Design review of the part built by this model. Coordinates are the model's own, in mm. A direction names the side the tool comes from. Give positions to 0.01 mm unless a question says otherwise; leave off trailing zeros. Order: outer loops, then holes, each group sorted by start corner. A loop starts at its lowest first (then second) coordinate and runs counter-clockwise, first axis right, second up. Notation, with made-up numbers: (-10, 40.5) -> (23, 40.5) arc R20 ccw to (23, 70.5) -> close; hole circle Ø8 at (60.5, 77). An arc over 180 degrees is marked (long way). One line per item, written item: value. Start each with the question number.
1) Consider section A-A (x = -49.5). State the section outline as (y, z) points, plus the area to 3 significant figures.
2) Consider section D-D (z = -28). State the section outline as (x, y) points.
3) For pin 1 (0.8 mm diameter, centred on x = -22.5, y = 1, fed in from +Z); pin 2 (0.8 mm diameter, centred on x = -45.5, y = 1, fed in from +Z); pin 3 (0.8 mm diameter, centred on x = -64.5, y = 0.5, fed in from -Z), all flat-tipped, find the tip position at first contact; note any pin that passes through.
4) Consider section C-C (z = -8). State the section outline as (x, y) points, plus the area to 3 significant figures.
5) Tool access review of faces 5 (the face through (-57, 1, -23.7)), 6 (the face through (-21.63, 0.811, -25.415)), 7 (the face through (-58, 1, -25.7)): name each direction out of +Z, -Z, +X, -X, +Y, -Y from which nothing blocks a thin tool from reaching the whole face with its end or side.
6) Wall thickness on line 1 along X through (y, z) = (1, -22); line 2 along Z through (x, y) = (-25, 0.45); line 3 along X through (y, z) = (0.1, 1): over which ranges is each line inside the solid? List them lowest first. Write a range as from..to.
7) Consider section B-B (z = -20.5). State the section outline as (x, y) points.
8) The part is to be moulded in two halves that separate along Z. For faces 1 (the face through (-68.93, 1, -13)), 2 (the face through (-60.915, 0.811, -10.199)), 3 (the face through (-45, 1, -30)), 4 (the face through (-43.43, 0.811, -15.985)), say which applies: released by +Z, released by -Z, zero draft, split by the parting line, or undercut.
from build123d import *

# Parameters (mm, degrees)
BOSS_EXTRUDE1_DEPTH = 1.6
FILLET1_R           = 1
FILLET2_R           = 1
FILLET3_R           = 0.2


with BuildPart() as part:
    # Sketch1 → Boss-Extrude1 (new body)
    with BuildSketch(Plane(origin=(0, 0, 0), x_dir=(1, 0, 0), z_dir=(0, 1, 0))):
        Polygon((-68.929583289, 0), (-64.629583289, 0), (-64.629583289, -1.3), (-65.129583289, -1.8), (-64.629583289, -2.3), (-63.629583289, -2.3), (-63.629583289, 0), (-61.629583289, 0), (-61.629583289, -2.3), (-60.629583289, -2.3), (-60.129583289, -1.8), (-60.629583289, -1.3), (-60.629583289, 0), (-60.129583289, 0), (-60.129583289, 5.5), (-45.129583289, 5.5), (-45.129583289, 7.5), (-60.629583289, 7.5), (-60.629583289, 10.5), (-65.329583289, 10.5), (-65.329583289, 11.9), (-60.629583289, 11.9), (-60.629583289, 14.7), (-65.329583289, 14.7), (-65.329583289, 23.7), (-47.129583289, 23.7), (-47.129583289, 15.7), (-45.129583289, 15.7), (-45.129583289, 30), (-47.129583289, 30), (-47.129583289, 25.7), (-68.929583289, 25.7), (-68.929583289, 20), align=None)
    boss_extrude1 = extrude(amount=BOSS_EXTRUDE1_DEPTH)

    # Mirror1: Boss-Extrude1 across plane
    add(boss_extrude1.mirror(Plane(origin=(-45.129583289, 1.6, -15.7), x_dir=(0, 0, 1), z_dir=(-1, 0, 0))))

    # Fillet1
    fillet1_edges = [part.edges().sort_by_distance(p)[0] for p in [
        (-68.929583289, 0.8, -25.7),
        (-47.129583289, 0.8, -25.7),
        (-47.129583289, 0.8, -30),
        (-47.129583289, 0.8, -15.7),
        (-47.129583289, 0.8, -23.7),
        (-21.329583289, 0.8, -25.7),
        (-43.129583289, 0.8, -25.7),
        (-43.129583289, 0.8, -30),
        (-43.129583289, 0.8, -15.7),
        (-43.129583289, 0.8, -23.7),
    ]]
    fillet(fillet1_edges, radius=FILLET1_R)

    # Fillet2
    fillet2_edges = [part.edges().sort_by_distance(p)[0] for p in [
        (-60.629583289, 0.8, -14.7),
        (-60.629583289, 0.8, -11.9),
        (-60.629583289, 0.8, -10.5),
        (-60.629583289, 0.8, -7.5),
        (-60.129583289, 0.8, -5.5),
        (-29.629583289, 0.8, -14.7),
        (-29.629583289, 0.8, -11.9),
        (-29.629583289, 0.8, -10.5),
        (-29.629583289, 0.8, -7.5),
        (-30.129583289, 0.8, -5.5),
    ]]
    fillet(fillet2_edges, radius=FILLET2_R)

    # Fillet3
    fillet3_edges = [part.edges().sort_by_distance(p)[0] for p in [
        (-60.629583289, 0.8, 1.3),
        (-60.129583289, 0.8, 1.8),
        (-60.629583289, 0.8, 2.3),
        (-61.629583289, 0.8, 2.3),
        (-63.629583289, 0.8, 2.3),
        (-64.629583289, 0.8, 2.3),
        (-65.129583289, 0.8, 1.8),
        (-64.629583289, 0.8, 1.3),
        (-29.629583289, 0.8, 1.3),
        (-30.129583289, 0.8, 1.8),
        (-29.629583289, 0.8, 2.3),
        (-28.629583289, 0.8, 2.3),
        (-26.629583289, 0.8, 2.3),
        (-25.629583289, 0.8, 2.3),
        (-25.129583289, 0.8, 1.8),
        (-25.629583289, 0.8, 1.3),
    ]]
    fillet(fillet3_edges, radius=FILLET3_R)


solid = part.part
Checked values:
1. outline: (0, -25.7) -> (1.6, -25.7) -> (1.6, -23.7) -> (0, -23.7) -> close; (0, -7.5) -> (1.6, -7.5) -> (1.6, -5.5) -> (0, -5.5) -> close
1. area: 6.40 mm^2
2. outline: (-47.13, 0) -> (-43.13, 0) -> (-43.13, 1.6) -> (-47.13, 1.6) -> close
3. pin 1: stops at z = 0
3. pin 2: stops at z = -5.5
3. pin 3: stops at z = -25.7
4. outline: (-68.93, 0) -> (-60.5, 0) -> (-60.5, 1.6) -> (-68.93, 1.6) -> close; (-29.76, 0) -> (-21.33, 0) -> (-21.33, 1.6) -> (-29.76, 1.6) -> close
4. area: 27.0 mm^2
5. face 5: +Y, -Y
5. face 6: -Z, +X, +Y, -Y
5. face 7: -Z, -X, +Y, -Y
6. line 1: x = -68.93..-65.33, -47.13..-43.13, -24.93..-21.33
6. line 2: z = -25.7..-23.7, -14.7..-11.9, -10.5..0
6. line 3: x = -64.63..-63.63, -61.63..-60.63, -29.63..-28.63, -26.63..-25.63
7. outline: (-68.93, 0) -> (-65.33, 0) -> (-65.33, 1.6) -> (-68.93, 1.6) -> close; (-47.13, 0) -> (-43.13, 0) -> (-43.13, 1.6) -> (-47.13, 1.6) -> close; (-24.93, 0) -> (-21.33, 0) -> (-21.33, 1.6) -> (-24.93, 1.6) -> close
8. face 1: zero draft
8. face 2: undercut
8. face 3: released by -Z
8. face 4: undercut
